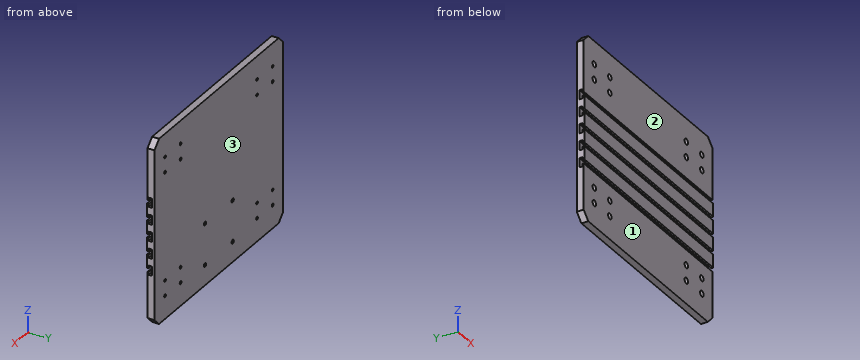
```python
from build123d import *

# Parameters (mm, degrees)
F0_W           = 355.6
F0_H           = 304.8
F1_DEPTH       = 12.7
F3_D           = 4.7752
F3_CBORE_D     = 9.525
F3_CBORE_DEPTH = 6.35
F5_DEPTH       = 355.601
F6_W           = 355.6
F6_H           = 97.79
F6_R           = 4.7625
F7_DEPTH       = 1.27
F8_W           = 355.6
F8_H           = 88.9
F8_R           = 4.7625
F9_DEPTH       = 1.27
F11_D          = 6.35
F11_DEPTH      = 6.35
F11_TIP        = 1.9077324654
F12_SIZE       = 12.7


with BuildPart() as f1:
    # F0 (on Front) → F1 (new body)
    with BuildSketch(Plane.XZ):
        with Locations((177.8, 152.4)):
            Rectangle(F0_W, F0_H)
    extrude(amount=F1_DEPTH)

    # F3 (through all)
    with Locations(Plane.XZ.offset(12.7)):
        with Locations((29.337, 266.7), (29.337, 241.3), (72.2122, 241.3), (72.2122, 266.7), (29.337, 63.5), (29.337, 38.1), (72.2122, 38.1), (72.2122, 63.5), (283.3624, 63.5), (283.3624, 38.1), (326.2376, 38.1), (326.2376, 63.5), (326.2376, 241.3), (283.3624, 241.3), (283.3624, 266.7), (326.2376, 266.7)):
            CounterBoreHole(F3_D / 2, F3_CBORE_D / 2, F3_CBORE_DEPTH)

    # F4 (on face) → F5 (cut, through all)
    with BuildSketch(Plane.YZ.offset(355.6)):
        Polygon((-9.525, 207.01), (-12.7, 207.01), (-12.7, 200.66), (-9.525, 200.66), (-9.525, 196.215), (-4.445, 196.215), (-4.445, 211.455), (-9.525, 211.455), align=None)
        Polygon((-12.7, 179.07), (-12.7, 172.72), (-9.525, 172.72), (-9.525, 168.275), (-4.445, 168.275), (-4.445, 183.515), (-9.525, 183.515), (-9.525, 179.07), align=None)
        Polygon((-12.7, 151.13), (-12.7, 144.78), (-9.525, 144.78), (-9.525, 140.335), (-4.445, 140.335), (-4.445, 155.575), (-9.525, 155.575), (-9.525, 151.13), align=None)
        Polygon((-12.7, 123.19), (-12.7, 116.8669015169), (-9.525, 116.84), (-9.525, 112.395), (-4.445, 112.395), (-4.445, 127.635), (-9.525, 127.635), (-9.525, 123.19), align=None)
        Polygon((-12.7, 95.25), (-12.7, 88.9), (-9.5218634233, 88.9), (-9.5218634233, 84.455), (-4.445, 84.455), (-4.445, 99.695), (-9.525, 99.695), (-9.525, 95.25), align=None)
    extrude(amount=-F5_DEPTH, mode=Mode.SUBTRACT)

    # F6 (on face) → F7 (cut)
    with BuildSketch(Plane.XZ.offset(12.7)):
        with Locations((177.8, 255.905)):
            Rectangle(F6_W, F6_H)
        with Locations((29.337, 241.3)):
            Circle(F6_R, mode=Mode.SUBTRACT)
        with Locations((72.2122, 241.3)):
            Circle(F6_R, mode=Mode.SUBTRACT)
        with Locations((283.3624, 241.3)):
            Circle(F6_R, mode=Mode.SUBTRACT)
        with Locations((326.2376, 241.3)):
            Circle(F6_R, mode=Mode.SUBTRACT)
        with Locations((29.337, 266.7)):
            Circle(F6_R, mode=Mode.SUBTRACT)
        with Locations((72.2122, 266.7)):
            Circle(F6_R, mode=Mode.SUBTRACT)
        with Locations((283.3624, 266.7)):
            Circle(F6_R, mode=Mode.SUBTRACT)
        with Locations((326.2376, 266.7)):
            Circle(F6_R, mode=Mode.SUBTRACT)
    extrude(amount=-F7_DEPTH, mode=Mode.SUBTRACT)

    # F8 (on face) → F9 (cut)
    with BuildSketch(Plane.XZ.offset(12.7)):
        with Locations((177.8, 44.45)):
            Rectangle(F8_W, F8_H)
        with Locations((29.337, 38.1)):
            Circle(F8_R, mode=Mode.SUBTRACT)
        with Locations((72.2122, 38.1)):
            Circle(F8_R, mode=Mode.SUBTRACT)
        with Locations((283.3624, 38.1)):
            Circle(F8_R, mode=Mode.SUBTRACT)
        with Locations((326.2376, 38.1)):
            Circle(F8_R, mode=Mode.SUBTRACT)
        with Locations((29.337, 63.5)):
            Circle(F8_R, mode=Mode.SUBTRACT)
        with Locations((72.2122, 63.5)):
            Circle(F8_R, mode=Mode.SUBTRACT)
        with Locations((283.3624, 63.5)):
            Circle(F8_R, mode=Mode.SUBTRACT)
        with Locations((326.2376, 63.5)):
            Circle(F8_R, mode=Mode.SUBTRACT)
    extrude(amount=-F9_DEPTH, mode=Mode.SUBTRACT)

    # F11
    with Locations(Plane(origin=(0, 0, 0), x_dir=(-1, 0, 0), z_dir=(0, 1, 0))):
        with Locations((-215.9, 101.6), (-215.9, 33.401), (-139.7, 33.401), (-139.7, 101.6)):
            Hole(F11_D / 2, depth=F11_DEPTH)
            with Locations((0, 0, -(F11_DEPTH + F11_TIP / 2))):  # 118° drill point
                Cone(0, F11_D / 2, F11_TIP, mode=Mode.SUBTRACT)

    # F12
    f12_edges = [f1.edges().sort_by_distance(p)[0] for p in [
        (355.6, -5.715, 304.8),
        (355.6, -5.715, 0),
        (0, -5.715, 304.8),
        (0, -5.715, 0),
    ]]
    chamfer(f12_edges, length=F12_SIZE)


solid = f1.part
```
Build history of the part. All positions in model axes, mm. Face numbers are marked on the shaded views. A direction names the side the tool comes from. Give positions to 0.01 mm unless a question says otherwise; leave off trailing zeros. Order: outer loops, then holes, each group sorted by start corner. A loop starts at its lowest first (then second) coordinate and runs counter-clockwise, first axis right, second up. Notation, with made-up numbers: M -7,10.5 L 35,10.5 A31 ccw 35,41.5 Z; hole C 80,6.25 d2. An arc over 180 degrees is marked long. Return JSON: item names as keys, results as strings.
Q1. 3-axis set-ups, long thin cutter, end or side, ignore diameter. For the marked faces 1, 2 and 3: which of +Z, -Z, +X, -X, +Y, -Y reach the whole face in a straight line?
Answer list:
{"face 1": "-Z, +X, -X, -Y", "face 2": "+Z, +X, -X, -Y", "face 3": "+Z, -Z, +X, -X, +Y"}
Q2. Band-saw the part on A-A (z = 283.5). Give the cut face in (x, y).
Answer list:
{"outline": "M 0,-11.43 L 355.6,-11.43 L 355.6,0 L 0,0 Z"}
Q3. Wall check: probe 1 along Z at (x, y) = (186.5, -4.75) (3 decimals); probe 2 along X at (y, z) = (-5, 266.7); probe 3 along X at (y, z) = (-9.3, 266.7). Give the ranges that are in metal, low to high. Write a range as from..to.
Answer list:
{"probe 1": "z = 0..84.455, 99.695..112.395, 127.635..140.335, 155.575..168.275, 183.515..196.215, 211.455..304.8", "probe 2": "x = 0..26.95, 31.72..69.82, 74.6..280.97, 285.75..323.85, 328.63..355.6", "probe 3": "x = 0..24.57, 34.1..67.45, 76.97..278.6, 288.12..321.48, 331..355.6"}
Q4. Flat gauge pins, fed straight in: pin 1 (5 mm diameter, centred on x = 165, z = 97, fed in from +Y); pin 2 (1 mm diameter, centred on x = 304.5, z = 229, fed in from -Y); pin 3 (5.5 mm diameter, centred on x = 72.21, z = 241.3, fed in from -Y). Where does each tip first touch, or does it go through?
Answer list:
{"pin 1": "stops at y = 0", "pin 2": "stops at y = -11.43", "pin 3": "stops at y = -6.35"}
